The drawing under review shows one solid part. Ordinate dimensions are in mm from its lowest x, y, z. A direction names the side the tool comes from. Round coordinates to 2 decimals unless told otherwise and drop trailing zeros. Write each loop counter-clockwise with the first axis right and the second up, starting at its lowest first coordinate (ties: lowest second). Pieces come first, ordered by that corner, then holes. Notation, with made-up numbers: M 2,24.5 L 13,24.5 A6 ccw 13,33.5 Z; hole C -4.5,16.25 d1. An arc over 180 degrees is marked long. Write item = value, one per line. Start each with the question number.
Item 1: Take a section at C-C, the plane y = 1.85. Give the number of separate pieces and of enclosed holes in the cut face, plus the area to 3 significant figures.
Item 2: Take a section at A-A, the plane x = 18. Give the boundary of the cut face in (y, z).
Item 3: Take a section at B-B, the plane z = 24.25. Give the boundary of the cut face in (x, y).
Item 4: To check wall thickness, follow line 1 along Z through (x, y) = (18, 1.5); line 2 along X through (y, z) = (1.3, 25.75) (1 decimal); line 3 along X through (y, z) = (1.9, 25) (1 decimal). State the ranges of each line that lie inside material, in increasing order.
Item 5: Take a section at D-D, the plane z = 27.5. Give the boundary of the cut face in (x, y), plus the area to 3 significant figures.
Item 6: Tool access review of the marked faces 4 and 5: name each direction out of +Z, -Z, +X, -X, +Y, -Y from which nothing blocks a thin tool from reaching the whole face with its end or side.
Item 7: For pin 1 Ø1 at (y, z) = (1.5, 11.5) entering from -X, flat-tipped, find the tip position at first contact; note if it passes through.
Item 8: The part is to be moulded in two halves that separate along X. For the marked faces 1, 2 and 3, say which applies: +X half, -X half, draft (parallel to the pull), parting line (faces both ways), or undercut.
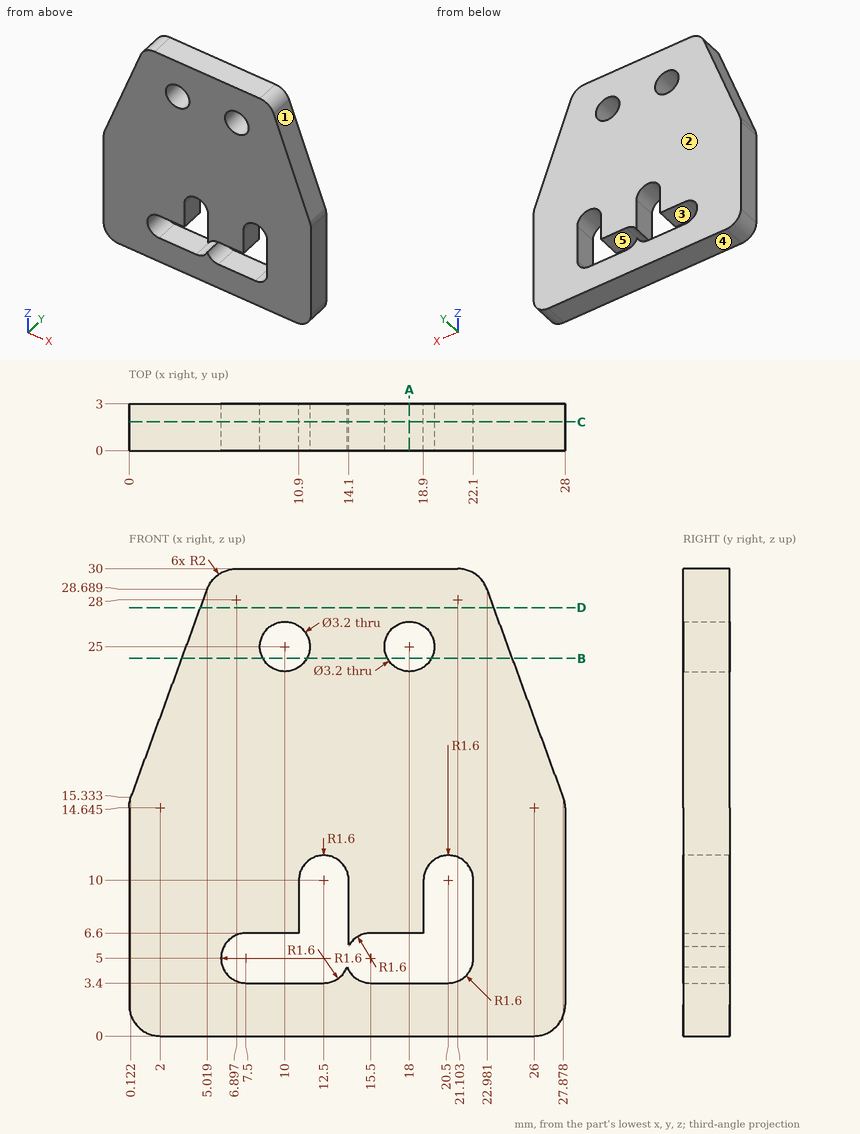
Response values:
q1.separate_pieces = 1
q1.enclosed_holes = 3
q1.area = 660 mm2
q2.outline = M 0,0 L 3,0 L 3,3.4 L 0,3.4 Z; M 0,6.6 L 3,6.6 L 3,23.4 L 0,23.4 Z; M 0,26.6 L 3,26.6 L 3,30 L 0,30 Z
q3.outline = M 3.39,0 L 8.59,0 L 8.59,3 L 3.39,3 Z; M 11.41,0 L 16.59,0 L 16.59,3 L 11.41,3 Z; M 19.41,0 L 24.61,0 L 24.61,3 L 19.41,3 Z
q4.line_1 = 0 to 3.4, 6.6 to 23.4, 26.6 to 30
q4.line_2 = 3.9 to 8.6, 11.4 to 16.6, 19.4 to 24.1
q4.line_3 = 3.7 to 8.4, 11.6 to 16.4, 19.6 to 24.3
q5.outline = M 4.58,0 L 23.42,0 L 23.42,3 L 4.58,3 Z
q5.area = 56.5 mm2
q6.face_4 = -Z, +X, -X, +Y, -Y
q6.face_5 = +Y, -Y
q7.pin_1 = 0
q8.face_1 = +X half
q8.face_2 = draft
q8.face_3 = undercut
